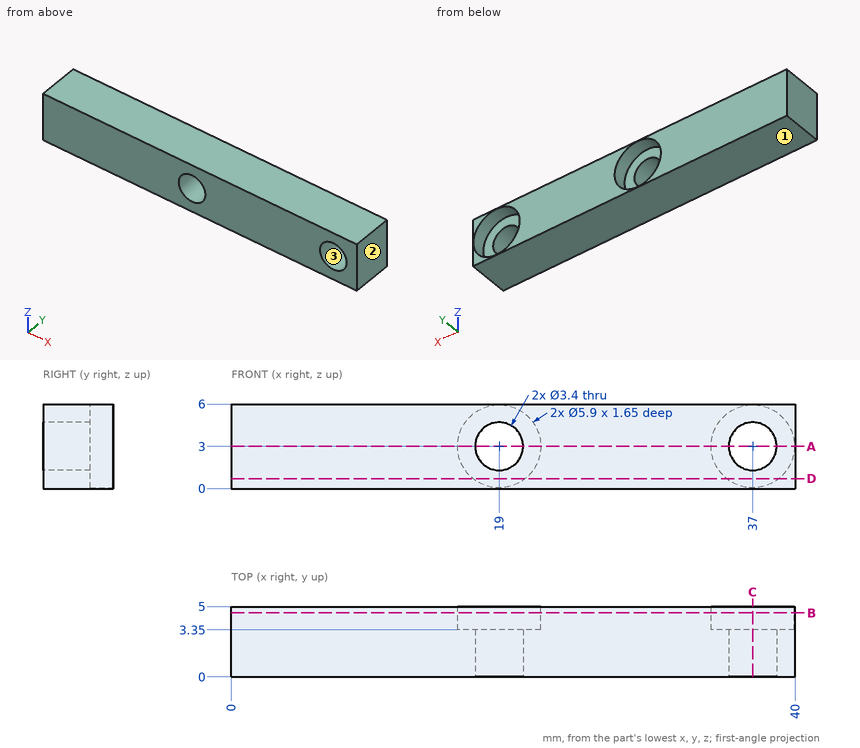
Study the drawing (mm; zero at the part's minimum x, y, z) and answer. Give positions to 0.01 mm unless a question says otherwise; leave off trailing zeros. Loops run counter-clockwise (first coordinate to the right, second up) from the corner with the lowest first, then second, coordinate; pieces in that order, holes last. Notation, with made-up numbers: (-8.5, 84) - (28.5, 84) arc R11 cw to (28.5, 96) - close; hole circle Ø3 at (-31.75, 24). An arc over 180 degrees is marked (long way). Answer as CSV lines item,"result". Start each with the question number.
1) Find section D-D (z = 0.7). Write down the section's boundary in (x, y), then the cut area to 3 significant figures.
2) Each of these flat-tipped pins is pushed along its axis until it touches: pin 1 Ø1 at (y, z) = (4.5, 5) entering from -X; pin 2 Ø1.8 at (x, z) = (17.5, 2.5) entering from +Y. Where does it stop, or does it pass through?
3) Find section B-B (y = 4.55). Write down the section's boundary in (x, z), then the cut area to 3 significant figures.
4) Determine the mould class of the marked faces 1, 2 and 3 for opening direction Z: released by +Z, released by -Z, zero draft, split by the parting line, or undercut.
5) Find section A-A (z = 3). Write down the section's boundary in (x, y).
6) Straight lines are drawn through the part: L1, parallel to Z at x = 19, y = 1.9; L2, parallel to X at y = 1.95, z = 2.8; L3, parallel to X at y = 0.95, z = 2.55. For each, find the intervals that lie inside material, in ascending order. Write a range as from..to.
7) Find section C-C (x = 37). Write down the section's boundary in (y, z), then the cut area to 4 significant figures.
Findings below:
1,outline,"(0, 0) - (40, 0) - (40, 5) - (38.85, 5) - (38.85, 3.35) - (35.15, 3.35) - (35.15, 5) - (20.85, 5) - (20.85, 3.35) - (17.15, 3.35) - (17.15, 5) - (0, 5) - close"
1,area,"188 mm^2"
2,pin 1,"x = 0"
2,pin 2,"y = 3.35"
3,outline,"(0, 0) - (40, 0) - (40, 6) - (0, 6) - close; hole circle Ø5.9 at (19, 3); hole circle Ø5.9 at (37, 3)"
3,area,"185 mm^2"
4,face 1,"released by -Z"
4,face 2,"zero draft"
4,face 3,"undercut"
5,outline,"(0, 0) - (17.3, 0) - (17.3, 3.35) - (16.05, 3.35) - (16.05, 5) - (0, 5) - close; (20.7, 0) - (35.3, 0) - (35.3, 3.35) - (34.05, 3.35) - (34.05, 5) - (21.95, 5) - (21.95, 3.35) - (20.7, 3.35) - close; (38.7, 0) - (40, 0) - (40, 5) - (39.95, 5) - (39.95, 3.35) - (38.7, 3.35) - close"
6,L1,"0..1.3, 4.7..6"
6,L2,"0..17.31, 20.69..35.31, 38.69..40"
6,L3,"0..17.36, 20.64..35.36, 38.64..40"
7,outline,"(0, 0) - (5, 0) - (5, 0.05) - (3.35, 0.05) - (3.35, 1.3) - (0, 1.3) - close; (0, 4.7) - (3.35, 4.7) - (3.35, 5.95) - (5, 5.95) - (5, 6) - (0, 6) - close"
7,area,"8.875 mm^2"
